```python
from build123d import *

# Parameters (mm, degrees)
F1_DEPTH = 25


with BuildPart() as f1:
    # F0 (on Front) → F1 (new body)
    with BuildSketch(Plane.XZ):
        with BuildLine():
            Line((32.5, 82.5), (-32.5, 82.5))
            Line((-32.5, 82.5), (-32.5, 78))
            ThreePointArc((-32.5, 78), (-31.328427, 75.171573), (-28.5, 74))
            Line((-28.5, 74), (-10.5, 74))
            ThreePointArc((-10.5, 74), (-4.843146, 71.656854), (-2.5, 66))
            Line((-2.5, 66), (-2.5, -66))
            ThreePointArc((-2.5, -66), (-4.843146, -71.656854), (-10.5, -74))
            Line((-10.5, -74), (-28.5, -74))
            ThreePointArc((-28.5, -74), (-31.328427, -75.171573), (-32.5, -78))
            Line((-32.5, -78), (-32.5, -82.5))
            Line((-32.5, -82.5), (32.5, -82.5))
            Line((32.5, -82.5), (32.5, -78))
            ThreePointArc((32.5, -78), (31.328427, -75.171573), (28.5, -74))
            Line((28.5, -74), (10.5, -74))
            ThreePointArc((10.5, -74), (4.843146, -71.656854), (2.5, -66))
            Line((2.5, -66), (2.5, 66))
            ThreePointArc((2.5, 66), (4.843146, 71.656854), (10.5, 74))
            Line((10.5, 74), (28.5, 74))
            ThreePointArc((28.5, 74), (31.328427, 75.171573), (32.5, 78))
            Line((32.5, 78), (32.5, 82.5))
        make_face()
    extrude(amount=F1_DEPTH)


solid = f1.part
```
The listing builds one solid part. Answer for the finished solid, in the listing's coordinates (mm). A direction names the side the tool comes from. Coordinates: 2 decimals unless noted, no trailing zeros. Write each loop counter-clockwise with the first axis right and the second up, starting at its lowest first coordinate (ties: lowest second). Pieces come first, ordered by that corner, then holes. Notation, with made-up numbers: M 80.5,59 L 116.5,59 A13 cw 116.5,63 Z; hole C 2,-16 d6. An arc over 180 degrees is marked long. Use a Markdown table: item, result. Add a question column.
1. For a pull along Z with two mould halves and no side action, classify faces 1 (the flat face through (0, -12, 82.5)), 2 (the flat face through (-19, -12, -74)), 3 (the flat face through (0, -25, 6)), 4 (the flat face through (0, -12, -82.5)) as +Z half, -Z half, draft (parallel to the pull), parting line (faces both ways), or undercut.
2. Straight lines are drawn through the part: line 1 along Z through (x, y) = (21.5, -17.75); line 2 along X through (y, z) = (-24, 48.5); line 3 along Z through (x, y) = (4, -4). For each, find the intervals that lie inside material, in ascending order. Write a range as [from, to].
3. Section B-B (y = -22.5) is taken. Give the vertices of the cut face in (x, z).
4. Section A-A (x = 7.5) is taken. Give the vertices of the cut face in (y, z).
5. Section D-D (z = -13) is taken. Give the vertices of the cut face in (x, y).
6. Given P1, Ø4, axis at y = -11.5, z = -4.5, coming from the -X side; P2, Ø8, axis at y = -16.5, z = -1, coming from the +X side, each flat-ended and moving along its own axis, determine where each tip first touches the part or whether it passes through.
7. Which of the six approach directions +Z, -Z, +X, -X, +Y, -Y give full straight-line access (tool end or side, diameter ignored) to faces 5 (the cylindrical face through (31.359, -12.325, -75.203)), 6 (the cylindrical face through (-4.906, -12.325, 71.719)), 7 (the flat face through (32.5, -12, 80))?
8. Section C-C (x = 21.5) is taken. Give the vertices of the cut face in (y, z), plus the area to 3 significant figures.
Data:
| question | item | result |
|---|---|---|
| 1 | face 1 | +Z half |
| 1 | face 2 | undercut |
| 1 | face 3 | draft |
| 1 | face 4 | -Z half |
| 2 | line 1 | z = [-82.5, -74], [74, 82.5] |
| 2 | line 2 | x = [-2.5, 2.5] |
| 2 | line 3 | z = [-82.5, -70.66], [70.66, 82.5] |
| 3 | outline | M -32.5,-82.5 L 32.5,-82.5 L 32.5,-78 A4 ccw 28.5,-74 L 10.5,-74 A8 cw 2.5,-66 L 2.5,66 A8 cw 10.5,74 L 28.5,74 A4 ccw 32.5,78 L 32.5,82.5 L -32.5,82.5 L -32.5,78 A4 ccw -28.5,74 L -10.5,74 A8 cw -2.5,66 L -2.5,-66 A8 cw -10.5,-74 L -28.5,-74 A4 ccw -32.5,-78 Z |
| 4 | outline | M -25,-82.5 L 0,-82.5 L 0,-73.42 L -25,-73.42 Z; M -25,73.42 L 0,73.42 L 0,82.5 L -25,82.5 Z |
| 5 | outline | M -2.5,-25 L 2.5,-25 L 2.5,0 L -2.5,0 Z |
| 6 | P1 | stops at x = -2.5 |
| 6 | P2 | stops at x = 2.5 |
| 7 | face 5 | +X, +Y, -Y |
| 7 | face 6 | -X, +Y, -Y |
| 7 | face 7 | +Z, -Z, +X, +Y, -Y |
| 8 | outline | M -25,-82.5 L 0,-82.5 L 0,-74 L -25,-74 Z; M -25,74 L 0,74 L 0,82.5 L -25,82.5 Z |
| 8 | area | 425 mm2 |
